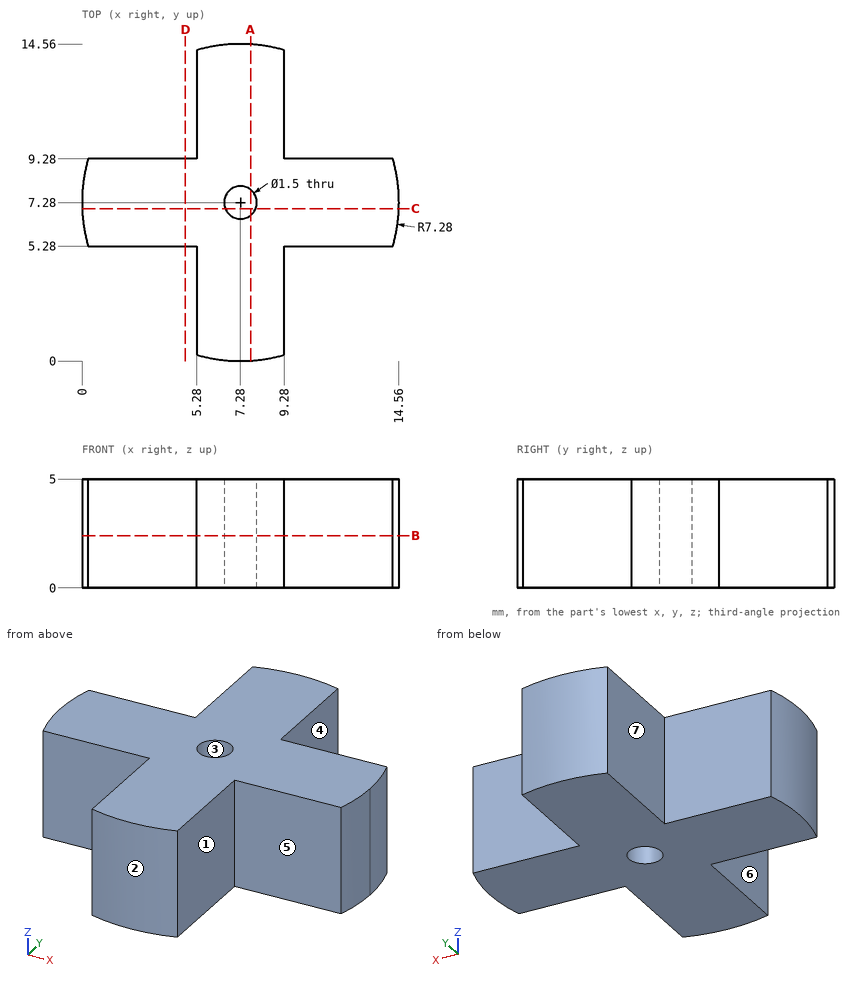
Answer from the drawing. Dimensions are ordinates in mm from the lowest x, y and z of the part. A direction names the side the tool comes from. Give positions to 0.01 mm unless a question says otherwise; leave off trailing zeros. Order: outer loops, then holes, each group sorted by start corner. A loop starts at its lowest first (then second) coordinate and runs counter-clockwise, first axis right, second up.
(1) Given pin 1 (2.5 mm diameter, centred on x = 12.5, z = 2, fed in from -Y); pin 2 (8 mm diameter, centred on x = 12.5, y = 9, fed in from -Z); pin 3 (2.5 mm diameter, centred on y = 13, z = 3.5, fed in from -X); pin 4 (2.5 mm diameter, centred on x = 11, z = 1.5, fed in from +Y), each flat-ended and moving along its own axis, determine where each tip first touches the part or whether it passes through.
(2) For the marked faces 4, 5, 6 and 7, determine the directions among +Z, -Z, +X, -X, +Y, -Y from which every point of the face is accessible in a straight line to the end or side of a thin tool.
(3) For a pull along Y with two mould halves and no side action, classify the marked faces 1, 2 and 3 as released by +Y, released by -Y, zero draft, split by the parting line, or undercut.
(4) Find section B-B (z = 2.4). Give the vertices of the cut face in (x, y).
(5) Find section C-C (y = 7). Give the vertices of the cut face in (x, z) (1 decimal), plus the area to 3 significant figures.
(6) Straight lines are drawn through the part: L1, parallel to X at y = 13, z = 2; L2, parallel to X at y = 8.75, z = 3.85. For each, find the intervals that lie inside material, in ascending order.
(7) Find section D-D (x = 4.75). Give the vertices of the cut face in (y, z).
(8) Find section A-A (x = 7.75). Give the vertices of the cut face in (y, z) (1 decimal), plus the area to 3 significant figures.
Result sheet:
1. pin 1: stops at y = 5.28
1. pin 2: stops at z = 0
1. pin 3: stops at x = 5.28
1. pin 4: stops at y = 9.28
2. face 4: +Z, -Z, +X, +Y
2. face 5: +Z, -Z, +X, -Y
2. face 6: +Z, -Z, -X, -Y
2. face 7: +Z, -Z, -X, +Y
3. face 1: zero draft
3. face 2: released by -Y
3. face 3: undercut
4. outline: (0.28, 5.28) - (5.28, 5.28) - (5.28, 0.28) arc R7.28 ccw to (9.28, 0.28) - (9.28, 5.28) - (14.28, 5.28) arc R7.28 ccw to (14.28, 9.28) - (9.28, 9.28) - (9.28, 14.28) arc R7.28 ccw to (5.28, 14.28) - (5.28, 9.28) - (0.28, 9.28) arc R7.28 ccw to start; hole circle Ø1.5 at (7.28, 7.28)
5. outline: (0, 0) - (6.6, 0) - (6.6, 5) - (0, 5) - close; (8, 0) - (14.6, 0) - (14.6, 5) - (8, 5) - close
5. area: 65.8 mm2
6. L1: x = 5.28 to 9.28
6. L2: x = 0.15 to 14.41
7. outline: (5.28, 0) - (9.28, 0) - (9.28, 5) - (5.28, 5) - close
8. outline: (0, 0) - (6.7, 0) - (6.7, 5) - (0, 5) - close; (7.9, 0) - (14.5, 0) - (14.5, 5) - (7.9, 5) - close
8. area: 66.8 mm2
